Input: part model. Units: mm. Frame: model coordinates. Coordinates: 2 decimals unless noted, no trailing zeros. Order: outer loops, then holes, each group sorted by start corner. A loop starts at its lowest first (then second) coordinate and runs counter-clockwise, first axis right, second up. Notation, with made-up numbers: M 36,7 L 72,7 A27 cw 72,33 Z; hole C -28.75,42 d1. An arc over 180 degrees is marked long. Answer in a Markdown table with one row per item.
Solid Edge part; units mm, degrees
sketch "Sketch1" plane through (0, 0, 0) normal (0, 0, 1) x (1, 0, 0)
  line L0 (400, 250) -> (-400, 250)
  line L1 (-400, 150) -> (-400, 250)
  line L2 (-50, 0) -> (-400, 150)
  arc A0 (50, 0) -> (-50, 0) centre (0, 0) cw
  line L3 (50, 0) -> (400, 150)
  line L4 (400, 150) -> (400, 250)
extrude "Protrusion1" add sketch "Sketch1" against normal blind 20
hole "Bohrung_1" at (0, 0, 0) direction (0, 0, -1) diameter 40 end up to next
hole "Bohrung_2" at (0, 0, 0) direction (0, 0, -1) diameter 52 depth 5
hole "Bohrung_3" at (-380, 230, 0) direction (0, 0, -1) diameter 11 end up to next start chamfer 1 start chamfer angle 45
hole "Hole1" at (-380, 170, 0) direction (0, 0, -1) diameter 11 end up to next start chamfer 1 start chamfer angle 45
hole "Hole2" at (380, 170, 0) direction (0, 0, -1) diameter 11 end up to next start chamfer 1 start chamfer angle 45
hole "Hole3" at (380, 230, 0) direction (0, 0, -1) diameter 11 end up to next start chamfer 1 start chamfer angle 45
hole "Bohrung_7" at (-300, 150, 0) direction (0, 0, -1) diameter 8.376 end up to next start chamfer 1 start chamfer angle 45
hole "Hole4" at (-250, 150, 0) direction (0, 0, -1) diameter 8.376 end up to next start chamfer 1 start chamfer angle 45
hole "Hole5" at (300, 150, 0) direction (0, 0, -1) diameter 8.376 end up to next start chamfer 1 start chamfer angle 45
hole "Hole6" at (250, 150, 0) direction (0, 0, -1) diameter 8.376 end up to next start chamfer 1 start chamfer angle 45
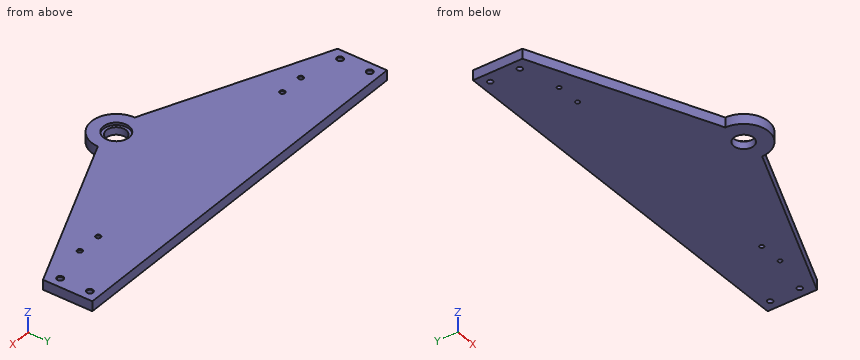
1) Cut plane B-B, the plane z = -16.5. State how many separate pieces and enclosed holes the cut face has, and give its area (3 significant figures).
Resolved:
| item | result |
|---|---|
| separate pieces | 1 |
| enclosed holes | 9 |
| area | 150,000 mm2 |
2) Cut plane D-D, the plane x = 346.5. Output: boundary loops of the cut face in (y, z).
Resolved:
| item | result |
|---|---|
| outline | M 127.07,-20 L 250,-20 L 250,0 L 127.07,0 Z |
3) Cut plane C-C, the plane y = 52.5. Output: boundary loops of the cut face in (x, z), and give its area (3 significant figures).
Resolved:
| item | result |
|---|---|
| outline | M -172.5,-20 L 172.5,-20 L 172.5,0 L -172.5,0 Z |
| area | 6,900 mm2 |
4) Cut plane A-A, the plane x = 0. Output: boundary loops of the cut face in (y, z).
Resolved:
| item | result |
|---|---|
| outline | M -50,-20 L -20,-20 L -20,-5 L -26,-5 L -26,0 L -50,0 Z; M 20,-20 L 250,-20 L 250,0 L 26,0 L 26,-5 L 20,-5 Z |
5) Material intervals for probe 1 along X at (y, z) = (150, -9.5); probe 2 along X at (y, z) = (231, -1.75); probe 3 along X at (y, z) = (0, -10.5), sorted ascending.
Resolved:
| item | result |
|---|---|
| probe 1 | x = -400 to -304.19, -295.81 to -254.19, -245.81 to 245.81, 254.19 to 295.81, 304.19 to 400 |
| probe 2 | x = -400 to -385.41, -374.59 to 374.59, 385.41 to 400 |
| probe 3 | x = -50 to -20, 20 to 50 |
6) Contact query for flat-ended pins moving along their axis: pin 1 (5 mm diameter, centred on y = 58.5, z = -18, fed in from +X); pin 2 (10 mm diameter, centred on y = 65.5, z = -15.5, fed in from +X); pin 3 (9.5 mm diameter, centred on x = -300, y = 150, fed in from -Z); pin 4 (5 mm diameter, centred on y = 0.5, z = -8.5, fed in from -X). Output: stop coordinate, or through.
Resolved:
| item | result |
|---|---|
| pin 1 | stops at x = 192.33 |
| pin 2 | stops at x = 214.5 |
| pin 3 | stops at z = -20 |
| pin 4 | stops at x = -57 |
